Check sheet for the drawn part. Datum: minimum x, y, z corner. Units: mm. A direction names the side the tool comes from. Round coordinates to 2 decimals unless told otherwise and drop trailing zeros. Order: outer loops, then holes, each group sorted by start corner. A loop starts at its lowest first (then second) coordinate and runs counter-clockwise, first axis right, second up. Notation, with made-up numbers: (-19.5, 56) -> (17.5, 56) arc R15 ccw to (17.5, 75) -> close; hole circle Ø4 at (74, 52.5). An arc over 180 degrees is marked (long way). Use CSV: the item, a comma, the result in double quotes.
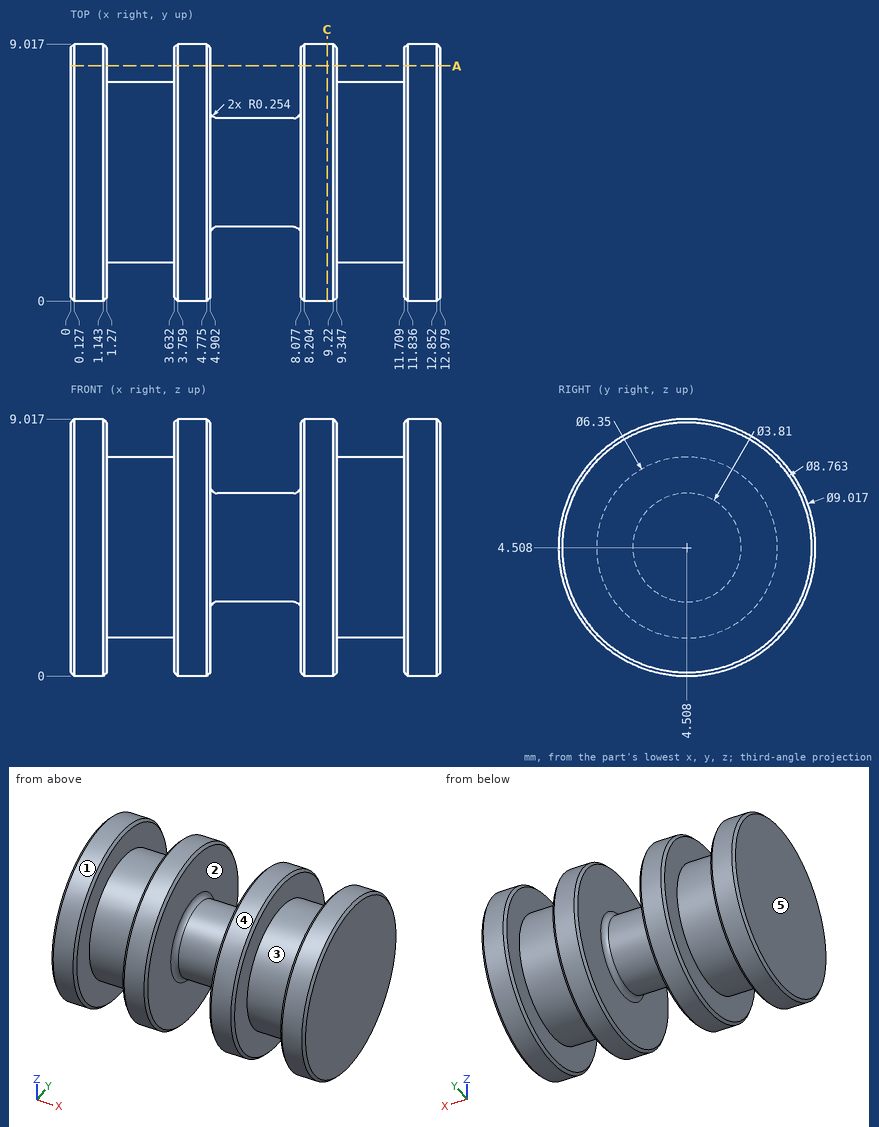
Q1. Scan lines: L1, parallel to X at y = 8.25, z = 6; L2, parallel to X at y = 4.75, z = 2; L3, parallel to Z at x = 1.5, y = 4.5. Record each from-to range of solid material in increasing order.
Result sheet:
L1,"x = 0 to 1.27, 3.63 to 4.9, 8.08 to 9.35, 11.71 to 12.98"
L2,"x = 0 to 4.9, 8.08 to 12.98"
L3,"z = 1.33 to 7.68"
Q2. Go/stop test with flat-tipped pins: pin 1 (1 mm diameter, centred on x = 4.5, y = 6.5, fed in from +Z); pin 2 (4 mm diameter, centred on x = 11.5, z = 7.5, fed in from -Y); pin 3 (3 mm diameter, centred on x = 6, y = 5.5, fed in from -Z); pin 4 (4.5 mm diameter, centred on y = 6.5, z = 5, fed in from -X). Record where each tip stops, or that it passes through.
Result sheet:
pin 1,"stops at z = 8.76"
pin 2,"stops at y = 0.12"
pin 3,"stops at z = 0"
pin 4,"stops at x = 0"
Q3. Access from +Z, -Z, +X, -X, +Y, -Y to the whole of each face (thin tool, end or side, straight path). Record for the marked faces 1 and 2.
Result sheet:
face 1,"+X, -X"
face 2,"none"
Q4. Sectioned sample at C-C, the plane x = 9. Enter the section's corners in (y, z).
Result sheet:
outline,"circle Ø9.02 at (4.51, 4.51)"
Q5. Mould release check, pull along X, two halves, no side actions. Record for the marked faces 3, 4 and 5: pulls with the +X half, pulls with the -X half, needs draft (parallel to the pull), parting line crosses it, or undercut.
Result sheet:
face 3,"undercut"
face 4,"needs draft"
face 5,"pulls with the -X half"
Q6. Sectioned sample at A-A, the plane y = 8.25. State how many separate pieces and enclosed holes the cut face has.
Result sheet:
separate pieces,"4"
enclosed holes,"0"
